```python
from build123d import *

# Parameters (mm, degrees)
CYLINDER002_R     = 3
CYLINDER002_DEPTH = 15
CYLINDER001_R     = 7.5
CYLINDER001_DEPTH = 1
CYLINDER_R        = 11.5
CYLINDER_DEPTH    = 40
SKETCH_R          = 1
POCKET_DEPTH      = 4
SKETCH001_R       = 23.34615
EXTRUDE_DEPTH     = 23


with BuildPart() as cylinder002:
    # Cylinder002 → Cylinder002 (new body)
    with BuildSketch(Plane.XY.offset(42)):
        Circle(CYLINDER002_R)
    extrude(amount=CYLINDER002_DEPTH)


with BuildPart() as cylinder001:
    # Cylinder001 → Cylinder001 (new body)
    with BuildSketch(Plane.XY.offset(41)):
        Circle(CYLINDER001_R)
    extrude(amount=CYLINDER001_DEPTH)


with BuildPart() as clone_of_pocket:
    # Cylinder → Cylinder (new body)
    with BuildSketch(Plane.XY.offset(1)):
        Circle(CYLINDER_R)
    extrude(amount=CYLINDER_DEPTH)

    # Fusion: union Cylinder002, Cylinder001
    add(cylinder002.part)
    add(cylinder001.part)

    # Sketch → Pocket (cut)
    with BuildSketch(Plane.XY.offset(41)):
        with Locations((8.227241, 4.75)):
            Circle(SKETCH_R)
        with Locations((-8.227241, 4.75)):
            Circle(SKETCH_R)
        with Locations((0, -9.5)):
            Circle(SKETCH_R)
    extrude(amount=-POCKET_DEPTH, mode=Mode.SUBTRACT)


with BuildPart() as common:
    # Sketch001 → Extrude (new body)
    with BuildSketch(Plane.XY.offset(41)):
        Circle(SKETCH001_R)
    extrude(amount=EXTRUDE_DEPTH)

    # Common: intersect Clone of Pocket
    add(clone_of_pocket.part, mode=Mode.INTERSECT)


solid = common.part
```
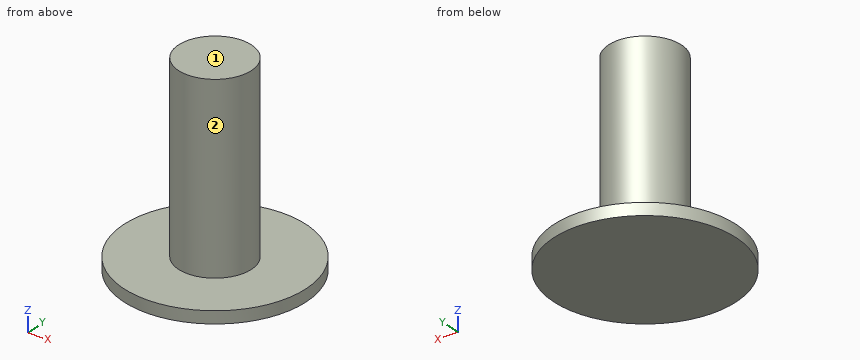
Build history of the part. All positions in model axes, mm. Face numbers are marked on the shaded views. A direction names the side the tool comes from. Give positions to 0.01 mm unless a question says otherwise; leave off trailing zeros. Order: outer loops, then holes, each group sorted by start corner. A loop starts at its lowest first (then second) coordinate and runs counter-clockwise, first axis right, second up. Notation, with made-up numbers: M -30.5,6 L -9.5,6 A21 ccw -9.5,21 Z; hole C 2,-8 d1. An arc over 180 degrees is marked long. Write item = value, one per line. Start each with the question number.
(1) Slice it at D-D on x = 3.5. Write the cut outline in (y, z).
(2) Probe L1, parallel to Z at x = -3, y = 6; L2, parallel to X at y = 2, z = 42.5; L3, parallel to Y at x = -1, z = 44.75. List the from-to ranges inside material, lowest first. Write a range as [from, to].
(3) Pin check, flat tips, straight feed: pin 1 Ø1.5 at (x, z) = (3, 44.5) entering from -Y; pin 2 Ø3 at (x, z) = (3.5, 53) entering from -Y; pin 3 Ø4 at (y, z) = (0.5, 48.5) entering from +X. Stop position of each tip, or through.
(4) Slice it at C-C on z = 47.5. Write the cut outline in (x, y).
(5) Slice it at A-A on y = 0. Write the cut outline in (x, z), plus the area to 3 significant figures.
(6) Which spindle directions (+Z, -Z, +X, -X, +Y, -Y) get a long thin tool onto all of the face, cutting with end or side? Do the marked faces 1 and 2. Say none if no direction does.
Responses:
q1.outline = M -6.63,41 L 6.63,41 L 6.63,42 L -6.63,42 Z
q2.L1 = [41, 42]
q2.L2 = [-2.24, 2.24]
q2.L3 = [-2.83, 2.83]
q3.pin_1 = -1.98
q3.pin_2 = -2.24
q3.pin_3 = 3
q4.outline = C 0,0 d6
q5.outline = M -7.5,41 L 7.5,41 L 7.5,42 L 3,42 L 3,57 L -3,57 L -3,42 L -7.5,42 Z
q5.area = 105 mm2
q6.face_1 = +Z, +X, -X, +Y, -Y
q6.face_2 = +Z
